For this review, take the finished solid that the model builds, in its own axes (mm). Coordinates: 2 decimals unless noted, no trailing zeros. Loops run counter-clockwise (first coordinate to the right, second up) from the corner with the lowest first, then second, coordinate; pieces in that order, holes last. Notation, with made-up numbers: (87, 71.5) -> (126, 71.5) arc R26 ccw to (126, 100.5) -> close; hole circle Ø9 at (87, -38). An arc over 180 degrees is marked (long way). Use a Markdown table: item, result.
from build123d import *

# Parameters (mm, degrees)
SKETCH1_W            = 15
SKETCH1_H            = 20
BOSS_EXTRUDE1_DEPTH  = 230
SKETCH2_W            = 65
SKETCH2_H            = 40
BOSS_EXTRUDE6_DEPTH  = 5
SKETCH7_W            = 75
SKETCH7_H            = 15
BOSS_EXTRUDE7_DEPTH  = 5
SKETCH8_W            = 75
SKETCH8_H            = 15
BOSS_EXTRUDE8_DEPTH  = 5
SKETCH9_W            = 65
SKETCH9_H            = 40
BOSS_EXTRUDE11_DEPTH = 5
CUT_EXTRUDE1_DEPTH   = 240.635139326
SKETCH13_R           = 1.984375
CUT_EXTRUDE2_DEPTH   = 10


with BuildPart() as part:
    # Sketch1 → Boss-Extrude1 (new body)
    with BuildSketch(Plane.XY):
        Rectangle(SKETCH1_W, SKETCH1_H)
    extrude(amount=BOSS_EXTRUDE1_DEPTH)

    # Sketch10 → Cut-Extrude1 (cut, through all)
    with BuildSketch(Plane.ZY.offset(7.5)):
        with BuildLine():
            Line((209.843145751, 2), (211.343145751, 2))
            ThreePointArc((211.343145751, 2), (223, 0), (211.343145751, -2))
            Line((211.343145751, -2), (209.843145751, -2))
            Line((209.843145751, -2), (209.843145751, 2))
        make_face()
    extrude(amount=-CUT_EXTRUDE1_DEPTH, mode=Mode.SUBTRACT)

    # Sketch13 → Cut-Extrude2 (cut)
    with BuildSketch(Plane(origin=(0, 10, 0), x_dir=(1, 0, 0), z_dir=(0, 1, 0))):
        with Locations(Location((0, -217, 0), (0, 0, 270))):
            Circle(SKETCH13_R)
    extrude(amount=-CUT_EXTRUDE2_DEPTH, mode=Mode.SUBTRACT)


with BuildPart() as body_2:
    # Sketch2 → Boss-Extrude6 (new body)
    with BuildSketch(Plane(origin=(0, 0, 0), x_dir=(-1, 0, 0), z_dir=(0, 0, -1))):
        with Locations((0, 30)):
            Rectangle(SKETCH2_W, SKETCH2_H)
    extrude(amount=-BOSS_EXTRUDE6_DEPTH)


with BuildPart() as body_3:
    # Sketch7 → Boss-Extrude7 (new body)
    with BuildSketch(Plane(origin=(32.5, 0, 0), x_dir=(0, 0, -1), z_dir=(1, 0, 0))):
        with Locations((-37.5, 30)):
            Rectangle(SKETCH7_W, SKETCH7_H)
    extrude(amount=BOSS_EXTRUDE7_DEPTH)


with BuildPart() as body_4:
    # Sketch8 → Boss-Extrude8 (new body)
    with BuildSketch(Plane.ZY.offset(32.5)):
        with Locations((37.5, 30)):
            Rectangle(SKETCH8_W, SKETCH8_H)
    extrude(amount=BOSS_EXTRUDE8_DEPTH)


with BuildPart() as body_5:
    # Sketch9 → Boss-Extrude11 (new body)
    with BuildSketch(Plane.XY.offset(75)):
        with Locations((0, 30)):
            Rectangle(SKETCH9_W, SKETCH9_H)
    extrude(amount=-BOSS_EXTRUDE11_DEPTH)


solid = part.part
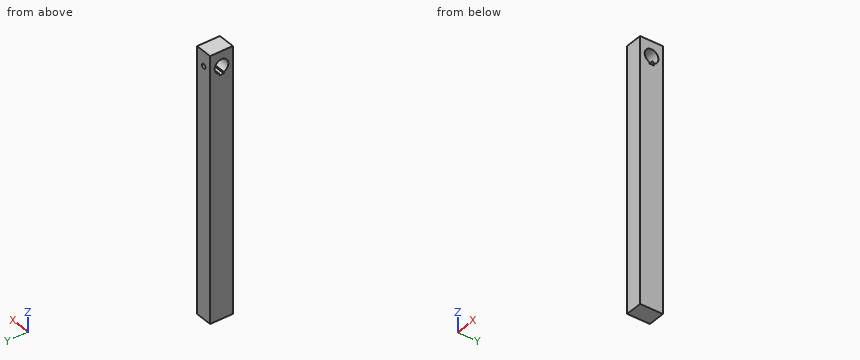
(1) Take a section at B-B on z = 217. Write out the cut boundary in (x, y).
Found:
| item | result |
|---|---|
| outline | (-7.5, -10) -> (7.5, -10) -> (7.5, -6) -> (-7.5, -6) -> close; (-7.5, 6) -> (-1.98, 6) -> (-1.98, 10) -> (-7.5, 10) -> close; (1.98, 6) -> (7.5, 6) -> (7.5, 10) -> (1.98, 10) -> close |
(2) For pin 1 Ø2.5 at (x, z) = (0, 217) entering from +Y; pin 2 Ø7 at (y, z) = (0, 217) entering from -X, all flat-tipped, find the tip position at first contact; note any pin that passes through.
Found:
| item | result |
|---|---|
| pin 1 | stops at y = -5.87 |
| pin 2 | passes through |
(3) Take a section at C-C on x = -5.25. Write out the cut boundary in (y, z), plus the area to 3 significant figures.
Found:
| item | result |
|---|---|
| outline | (-10, 0) -> (10, 0) -> (10, 230) -> (-10, 230) -> close; hole (-2, 209.84) -> (2, 209.84) -> (2, 211.34) arc R6 ccw (long way) to (-2, 211.34) -> close |
| area | 4,480 mm^2 |
(4) For line 1 along X through (y, z) = (7.65, 217); line 2 along Z through (x, y) = (0, 7.4); line 3 along Z through (x, y) = (-1.25, -0.25), list the stretches that pass through material, from the lowest coordinate up.
Found:
| item | result |
|---|---|
| line 1 | x = -7.5 to -1.98, 1.98 to 7.5 |
| line 2 | z = 0 to 215.02, 218.98 to 230 |
| line 3 | z = 0 to 209.84, 222.99 to 230 |
(5) Take a section at A-A on y = 0. Write out the cut boundary in (x, z).
Found:
| item | result |
|---|---|
| outline | (-7.5, 0) -> (7.5, 0) -> (7.5, 209.84) -> (-7.5, 209.84) -> close; (-7.5, 223) -> (7.5, 223) -> (7.5, 230) -> (-7.5, 230) -> close |
